Work out the finished part from the listing and answer in its coordinate system (mm). Face numbers are marked on the shaded views. A direction names the side the tool comes from. Coordinates: 2 decimals unless noted, no trailing zeros. Write each loop counter-clockwise with the first axis right and the second up, starting at its lowest first coordinate (ties: lowest second). Pieces come first, ordered by that corner, then holes. Notation, with made-up numbers: (25, 58.25) - (73, 58.25) arc R20 ccw to (73, 85.25) - close; hole circle Ø7 at (-5.5, 25.25). An arc over 180 degrees is marked (long way). Answer as a JSON object with one key per item and string values. Group by question number.
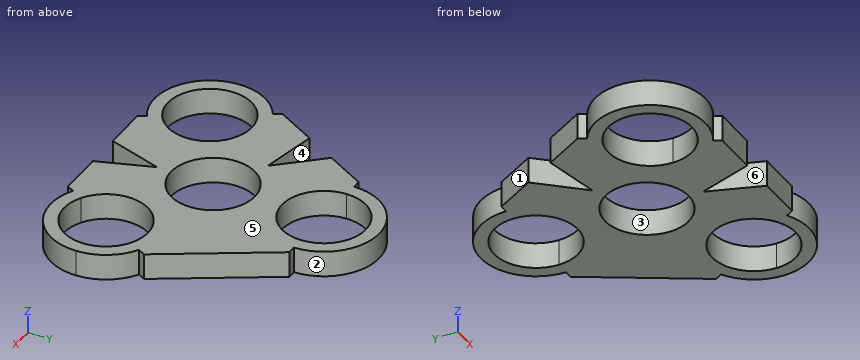
from build123d import *

# Parameters (mm, degrees)
F0_R     = 11.35
F1_DEPTH = 7
F3_DEPTH = 50.7


# Not quite as in the source:
# - a feature names something its author has since deleted; it is built from what else it names


with BuildPart() as f1:
    # F0 (on Top) → F1 (new body)
    with BuildSketch(Plane.XY):
        with BuildLine():
            Line((-31.5669890957, -5.0726587053), (-33.3938997814, -1.9127698865))
            ThreePointArc((-33.3938997814, -1.9127698865), (-38.8718921093, -22.4064664798), (-18.378195516, -27.8844588077))
            Line((-18.378195516, -27.8844588077), (-20.2051062016, -24.7245699889))
            ThreePointArc((-20.2051062016, -24.7245699889), (-35.7120032905, -20.5795557942), (-31.5669890957, -5.0726587053))
        make_face()
        with BuildLine():
            ThreePointArc((-10.8860476487, -14.8986143471), (-18.3899747432, -1.9059667726), (-33.3938997814, -1.9127698865))
            Line((-33.3938997814, -1.9127698865), (-31.5669890957, -5.0726587053))
            ThreePointArc((-31.5669890957, -5.0726587053), (-20.2140191502, -5.0675110157), (-14.5360476487, -14.8986143471))
            ThreePointArc((-14.5360476487, -14.8986143471), (-16.0549443173, -20.5706428456), (-20.2051062016, -24.7245699889))
            Line((-20.2051062016, -24.7245699889), (-18.378195516, -27.8844588077))
            ThreePointArc((-18.378195516, -27.8844588077), (-12.8934000742, -22.3946872526), (-10.8860476487, -14.8986143471))
        make_face()
        with BuildLine():
            ThreePointArc((-11.3499979258, 29.9931382104), (-0.0068617896, 41.3499979258), (11.3499979258, 30.0068617896))
            Line((11.3499979258, 30.0068617896), (14.9999972588, 30.0090684445))
            ThreePointArc((14.9999972588, 30.0090684445), (-0.0090684445, 44.9999972588), (-14.9999972588, 29.9909315555))
            Line((-14.9999972588, 29.9909315555), (-11.3499979258, 29.9931382104))
        make_face()
        with BuildLine():
            ThreePointArc((11.3499979258, 30.0068617896), (11.3499994815, 30.003430895), (11.35, 30))
            ThreePointArc((11.35, 30), (0.003430895, 18.6500005185), (-11.3499979258, 29.9931382104))
            Line((-11.3499979258, 29.9931382104), (-14.9999972588, 29.9909315555))
            ThreePointArc((-14.9999972588, 29.9909315555), (0.0045342224, 15.0000006853), (15, 30))
            ThreePointArc((15, 30), (14.9999993147, 30.0045342224), (14.9999972588, 30.0090684445))
            Line((14.9999972588, 30.0090684445), (11.3499979258, 30.0068617896))
        make_face()
        with BuildLine():
            Line((31.6093732737, -5.0344646094), (33.4324619211, -1.8723691359))
            ThreePointArc((33.4324619211, -1.8723691359), (12.9454038899, -7.3751369148), (18.4481716689, -27.8621949459))
            Line((18.4481716689, -27.8621949459), (20.2712603162, -24.7000994724))
            ThreePointArc((20.2712603162, -24.7000994724), (16.1074993635, -9.1982255621), (31.6093732737, -5.0344646094))
        make_face()
        with BuildLine():
            ThreePointArc((40.940316795, -14.8672820409), (38.928430147, -7.3633556317), (33.4324619211, -1.8723691359))
            Line((33.4324619211, -1.8723691359), (31.6093732737, -5.0344646094))
            ThreePointArc((31.6093732737, -5.0344646094), (35.7679892314, -9.189311058), (37.290316795, -14.8672820409))
            ThreePointArc((37.290316795, -14.8672820409), (31.6182877779, -24.6949544773), (20.2712603162, -24.7000994724))
            Line((20.2712603162, -24.7000994724), (18.4481716689, -27.8621949459))
            ThreePointArc((18.4481716689, -27.8621949459), (33.4442432041, -27.855395393), (40.940316795, -14.8672820409))
        make_face()
        with BuildLine():
            Line((17.2754548146, 30.0104441021), (14.9999972588, 30.0090684445))
            ThreePointArc((14.9999972588, 30.0090684445), (14.9999993147, 30.0045342224), (15, 30))
            ThreePointArc((15, 30), (0.0045342224, 15.0000006853), (-14.9999972588, 29.9909315555))
            Line((-14.9999972588, 29.9909315555), (-17.2754548146, 29.9895558979))
            Line((-17.2754548146, 29.9895558979), (-34.5328199137, 0.0571463332))
            Line((-34.5328199137, 0.0571463332), (-33.3938997814, -1.9127698865))
            ThreePointArc((-33.3938997814, -1.9127698865), (-18.3899747432, -1.9059667726), (-10.8860476487, -14.8986143471))
            ThreePointArc((-10.8860476487, -14.8986143471), (-12.8934000742, -22.3946872526), (-18.378195516, -27.8844588077))
            Line((-18.378195516, -27.8844588077), (-17.2392753837, -29.8543750274))
            Line((-17.2392753837, -29.8543750274), (17.3116342454, -29.8334868233))
            Line((17.3116342454, -29.8334868233), (18.4481716689, -27.8621949459))
            ThreePointArc((18.4481716689, -27.8621949459), (12.9454038899, -7.3751369148), (33.4324619211, -1.8723691359))
            Line((33.4324619211, -1.8723691359), (34.5689993445, 0.0989227415))
            Line((34.5689993445, 0.0989227415), (17.2754548146, 30.0104441021))
        make_face()
        Circle(F0_R, mode=Mode.SUBTRACT)
    extrude(amount=F1_DEPTH)

    # F2 (on face) → F3 (cut)
    with BuildSketch(Plane.XY.offset(7)):
        Polygon((-13.1224627256, 7.654147332), (-23.4067556554, 19.3549887506), (-28.4015190728, 10.6917134805), align=None)
        Polygon((-0.067454671, -15.1914597466), (-5.0242557701, -29.8469902776), (4.9070631834, -29.8409861689), align=None)
    extrude(amount=-F3_DEPTH, mode=Mode.SUBTRACT)


solid = f1.part
Q1. Section A-A on x = -25 is taken. Determine the outline of the cut face in (y, z), plus the area to 3 significant figures.
Q2. Section C-C on y = -7 is taken. Determine the outline of the cut face in (x, z), plus the area to 3 significant figures.
Q3. Section B-B on z = 1.5 is taken. Count the separate pieces of the cut face and the enclosed holes in it, plus the area to 3 significant figures.
Q4. For a pull along X with two mould halves and no side action, classify the marked faces 1, 2 and 3 as +X half, -X half, draft (parallel to the pull), parting line (faces both ways), or undercut.
Q5. Consider L1, parallel to X at y = -14.5, z = 2.25; L2, parallel to X at y = -12, z = 2.75; L3, parallel to Y at x = 36, z = 2. Determine where each line is inside the solid, lowest interval first. Write a range as from..to.
Q6. Section D-D on x = -1.5 is taken. Determine the outline of the cut face in (y, z), plus the area to 3 significant figures.
Q7. Flat-ended cylindrical pins translate along their axes: pin 1 Ø3 at (y, z) = (19, 4) entering from +X; pin 2 Ø2 at (x, z) = (21, 5) entering from -Y; pin 3 Ø1.5 at (x, z) = (-28.5, 1) entering from +Y; pin 4 Ø20.5 at (x, y) = (0, 0) entering from -Z. Find the tip coordinate at first contact, or state that the pin passes through.
Q8. A tool of negligible diameter and unlimited length cuts with its end or side. For the marked faces 4, 5 and 6, from which of +Z, -Z, +X, -X, +Y, -Y can it reach the whole face along a straight path? Write none if from no direction.
Numbers:
{
 "1": {"outline": "(-29.87, 0) - (-26.21, 0) - (-26.21, 7) - (-29.87, 7) - close; (-3.58, 0) - (10.02, 0) - (10.02, 7) - (-3.58, 7) - close", "area": "121 mm²"},
 "2": {"outline": "(-38.64, 0) - (-34.04, 0) - (-34.04, 7) - (-38.64, 7) - close; (-17.74, 0) - (-8.93, 0) - (-8.93, 7) - (-17.74, 7) - close; (8.93, 0) - (17.76, 0) - (17.76, 7) - (8.93, 7) - close; (34.12, 0) - (38.71, 0) - (38.71, 7) - (34.12, 7) - close", "area": "188 mm²"},
 "3": {"separate pieces": "1", "enclosed holes": "4", "area": "2,400 mm²"},
 "4": {"face 1": "-X half", "face 2": "parting line", "face 3": "undercut"},
 "5": {"L1": "x = -40.88..-37.23, -14.54..14.6, 37.28..40.94", "L2": "x = -40.6..-36.86, -14.91..14.96, 36.92..40.66", "L3": "y = -25.99..-20.12, -9.61..-3.74"},
 "6": {"outline": "(-19.43, 0) - (-11.25, 0) - (-11.25, 7) - (-19.43, 7) - close; (11.25, 0) - (18.75, 0) - (18.75, 7) - (11.25, 7) - close; (41.25, 0) - (44.92, 0) - (44.92, 7) - (41.25, 7) - close", "area": "135 mm²"},
 "7": {"pin 1": "stops at x = 24.51", "pin 2": "stops at y = -29.34", "pin 3": "stops at y = 10.69", "pin 4": "passes through"},
 "8": {"face 4": "+Z, -Z", "face 5": "+Z, +X, -X, +Y, -Y", "face 6": "+Z, -Z, -Y"}
}
